The listing builds one solid part. Answer for the finished solid, in the listing's coordinates (mm). Face numbers are marked on the shaded views. Coordinates: 2 decimals unless noted, no trailing zeros. Order: outer loops, then holes, each group sorted by start corner. A loop starts at its lowest first (then second) coordinate and runs counter-clockwise, first axis right, second up. Notation, with made-up numbers: (79, 44) - (97, 44) arc R35 cw to (97, 82) - close; hole circle Ø2 at (88.25, -30). An arc over 180 degrees is marked (long way). One line per item, written item: value. Start each with the question number.
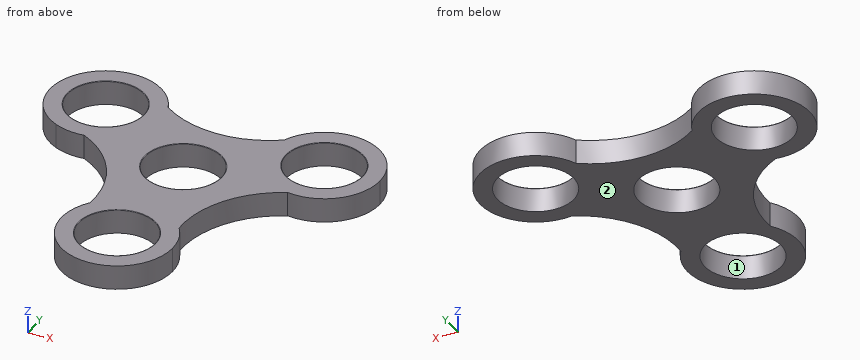
```python
from build123d import *

# Parameters (mm, degrees)
F0_R     = 11
F1_DEPTH = 7
F2_DEPTH = 7
F3_R     = 0.15
F4_R     = 0.15
F5_R     = 0.15


# Not quite as in the source:
# - a feature names something its author has since deleted; it is built from what else it names


with BuildPart() as f1:
    # F0 (on Top) → F1 (new body)
    with BuildSketch(Plane.XY):
        with BuildLine():
            ThreePointArc((29.3501442774, 1.4728811124), (17.7035935394, 9.3195381001), (16.7314646223, 23.3290753994))
            ThreePointArc((16.7314646223, 23.3290753994), (0, 18.0157402468), (-16.7314646223, 23.3290753994))
            ThreePointArc((-16.7314646223, 23.3290753994), (-15.8555966996, 20.3808641164), (-15.56, 17.3195381001))
            ThreePointArc((-15.56, 17.3195381001), (-19.4902507988, 6.8161503505), (-29.3501442774, 1.4728811124))
            ThreePointArc((-29.3501442774, 1.4728811124), (-16.8351135056, -10.0081099666), (-12.8952216464, -26.5282916699))
            ThreePointArc((-12.8952216464, -26.5282916699), (-0.0001071921, -20.0000000004), (12.8950947338, -26.5281188876))
            ThreePointArc((12.8950947338, -26.5281188876), (16.8350899961, -10.0080120701), (29.3501442774, 1.4728811124))
        make_face()
        Circle(F0_R, mode=Mode.SUBTRACT)
    extrude(amount=F1_DEPTH)

    # F0 (on Top) → F2 (join)
    with BuildSketch(Plane.XY):
        with BuildLine():
            ThreePointArc((29.3501442774, 1.4728811124), (42.0633877496, 5.2497888988), (47.56, 17.3195381001))
            ThreePointArc((47.56, 17.3195381001), (34.6213260163, 33.0239414005), (16.7314646223, 23.3290753994))
            ThreePointArc((16.7314646223, 23.3290753994), (17.7035935394, 9.3195381001), (29.3501442774, 1.4728811124))
        make_face()
        with Locations((31.56, 17.3195381001)):
            Circle(F0_R, mode=Mode.SUBTRACT)
        with BuildLine():
            ThreePointArc((-15.56, 17.3195381001), (-15.8555966996, 20.3808641164), (-16.7314646223, 23.3290753994))
            ThreePointArc((-16.7314646223, 23.3290753994), (-42.6554805123, 28.8473441446), (-38.1316823001, 2.7314267848))
            ThreePointArc((-38.1316823001, 2.7314267848), (-33.8298826127, 1.4813679746), (-29.3501442774, 1.4728811124))
            ThreePointArc((-29.3501442774, 1.4728811124), (-19.4902507988, 6.8161503505), (-15.56, 17.3195381001))
        make_face()
        with Locations((-31.56, 17.3195381001)):
            Circle(F0_R, mode=Mode.SUBTRACT)
        with BuildLine():
            ThreePointArc((16, -36), (15.2039717794, -31.0161017135), (12.8950947338, -26.5281188876))
            ThreePointArc((12.8950947338, -26.5281188876), (-0.0001071921, -20.0000000004), (-12.8952216464, -26.5282916699))
            ThreePointArc((-12.8952216464, -26.5282916699), (-4.9837964273, -51.2040051687), (16, -36))
        make_face()
        with Locations((0, -36)):
            Circle(F0_R, mode=Mode.SUBTRACT)
    extrude(amount=F2_DEPTH)

    # F3
    f3_edges = [f1.edges().sort_by_distance(p)[0] for p in [
        (-11, 0, 7),
    ]]
    fillet(f3_edges, radius=F3_R)

    # F4
    f4_edges = [f1.edges().sort_by_distance(p)[0] for p in [
        (-42.56, 17.319538, 7),
        (-11, -36, 7),
    ]]
    fillet(f4_edges, radius=F4_R)

    # F5
    f5_edges = [f1.edges().sort_by_distance(p)[0] for p in [
        (20.56, 17.319538, 7),
    ]]
    fillet(f5_edges, radius=F5_R)


solid = f1.part
```
(1) Consider probe 1 along Y at (x, z) = (0, 3.5); probe 2 along Y at (x, z) = (31.56, 2); probe 3 along Y at (x, z) = (-3, 1.5). Determine where each line is inside the solid, lowest interval first.
(2) Flat-ended cylindrical pins translate along their axes: pin 1 Ø4 at (y, z) = (-2.5, 5.5) entering from -X; pin 2 Ø20 at (x, y) = (-31.56, 17.32) entering from +Z; pin 3 Ø2 at (y, z) = (-39, 1.5) entering from +X; pin 4 Ø1.5 at (x, z) = (17, 2.5) entering from +Y. Find the tip coordinate at first contact, or state that the pin passes through.
(3) The part is cut by section A-A on x = 0. Determine the outline of the cut face in (y, z).
(4) The part is cut by section C-C on z = 3.75. Determine the outline of the cut face in (x, y), plus the area to 3 significant figures.
(5) For a pull along X with two mould halves and no side action, classify the marked faces 1 and 2 as pulls with the +X half, pulls with the -X half, needs draft (parallel to the pull), parting line crosses it, or undercut.
(6) The part is cut by section B-B on x = -31.56. Determine the outline of the cut face in (y, z).
(7) The part is cut by section D-D on y = 0. Determine the outline of the cut face in (x, z).
Completed:
1. probe 1: y = -52 to -47, -25 to -11, 11 to 18.02
1. probe 2: y = 1.32 to 6.32, 28.32 to 33.32
1. probe 3: y = -51.72 to -46.58, -25.42 to -10.58, 10.58 to 18.17
2. pin 1: stops at x = -25.86
2. pin 2: passes through
2. pin 3: stops at x = 15.87
2. pin 4: stops at y = 25.4
3. outline: (-52, 0) - (-47, 0) - (-47, 6.85) arc R0.15 ccw to (-47.15, 7) - (-52, 7) - close; (-25, 0) - (-11, 0) - (-11, 6.85) arc R0.15 ccw to (-11.15, 7) - (-24.85, 7) arc R0.15 ccw to (-25, 6.85) - close; (11, 0) - (18.02, 0) - (18.02, 7) - (11.15, 7) arc R0.15 ccw to (11, 6.85) - close
4. outline: (-29.35, 1.47) arc R29 cw to (-12.9, -26.53) arc R16 ccw (long way) to (12.9, -26.53) arc R29 cw to (29.35, 1.47) arc R16 ccw (long way) to (16.73, 23.33) arc R29 cw to (-16.73, 23.33) arc R16 ccw (long way) to start; hole circle Ø22 at (-31.56, 17.32); hole circle Ø22 at (0, -36); hole circle Ø22 at (0, 0); hole circle Ø22 at (31.56, 17.32)
4. area: 2,410 mm2
5. face 1: undercut
5. face 2: needs draft
6. outline: (1.32, 0) - (6.32, 0) - (6.32, 6.85) arc R0.15 ccw to (6.17, 7) - (1.32, 7) - close; (28.32, 0) - (33.32, 0) - (33.32, 7) - (28.47, 7) arc R0.15 ccw to (28.32, 6.85) - close
7. outline: (-26.64, 0) - (-11, 0) - (-11, 6.85) arc R0.15 ccw to (-11.15, 7) - (-26.64, 7) - close; (11, 0) - (26.64, 0) - (26.64, 7) - (11.15, 7) arc R0.15 ccw to (11, 6.85) - close
